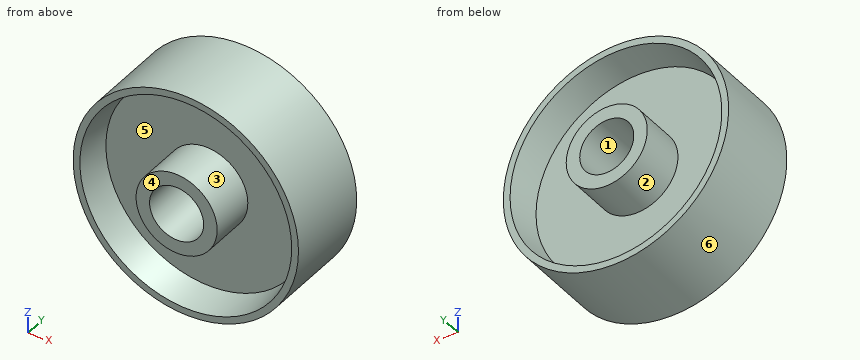
Autodesk Inventor part; units mm, degrees
ref_plane "YZ Plane" through (0, 0, 0) normal (1, 0, 0) x (0, 1, 0)
ref_plane "XZ Plane" through (0, 0, 0) normal (0, 1, 0) x (-1, 0, 0)
ref_plane "XY Plane" through (0, 0, 0) normal (0, 0, 1) x (1, 0, 0)
sketch "Sketch1" plane through (0, 0, 0) normal (0, 0, 1) x (1, 0, 0)
  line L0 (0, 40) -> (0, -30)
  line L1 (8.2, 0) -> (61.4, 0)
  line L2 (12, 25) -> (12, -25)
  line L3 (12, 25) -> (18, 25)
  line L4 (18, 25) -> (18, 5)
  line L5 (18, 5) -> (45, 5)
  line L6 (47, 19) -> (50, 19)
  line L7 (50, 19) -> (50, -19)
  line L8 (50, -19) -> (47, -19)
  line L9 (47, -19) -> (45, -5)
  line L10 (45, -5) -> (18, -5)
  line L11 (18, -5) -> (18, -25)
  line L12 (18, -25) -> (12, -25)
  line L13 (45, 5) -> (47, 19)
  dimension "d0" = 50
  dimension "d1" = 24
  dimension "d2" = 36
  dimension "d3" = 100
  dimension "d4" = 3
  dimension "d5" = 10
  dimension "d6" = 5
  dimension "d7" = 38
revolve "Revolution1" add sketch "Sketch1" angle 360 about axis through (0, 0, 0) along (0, -1, 0)
properties part number "Wheel" material "Thermoplastic Resin"
Design review of the part built by this model. Coordinates are the model's own, in mm. Face numbers are marked on the shaded views. A direction names the side the tool comes from. Round coordinates to 2 decimals unless told otherwise and drop trailing zeros. Write each loop counter-clockwise with the first axis right and the second up, starting at its lowest first coordinate (ties: lowest second). Pieces come first, ordered by that corner, then holes. Notation, with made-up numbers: (8, 82) - (43, 82) arc R27 ccw to (43, 100) - close; hole circle Ø3 at (53.5, 20.5). An arc over 180 degrees is marked (long way). Return JSON: item names as keys, results as strings. Group by question number.
Item 1: For probe 1 along Z at (x, y) = (0, 4.5); probe 2 along X at (y, z) = (-18.5, 1.5); probe 3 along X at (y, z) = (20.5, 0.5), list the stretches that pass through material, from the lowest coordinate up. Write a range as [from, to].
Item 2: We need section D-D on y = 22.5. Write out the cut boundary in (x, z), and give its area (3 significant figures).
Item 3: Insertion check: P1, Ø3, axis at x = 38.5, z = -36.5, coming from the +Y side; P2, Ø10, axis at x = -11.5, y = 7, coming from the -Z side; P3, Ø8, axis at x = -38.5, z = -36.5, coming from the +Y side; P4, Ø8, axis at x = 17.5, z = -24, coming from the -Y side. Each pin has a flat end and moves straight along its axis. Give the tip position at first contact, or say it passes through.
Item 4: We need section B-B on x = 0. Write out the cut boundary in (y, z).
Item 5: We need section A-A on z = 0. Write out the cut boundary in (x, y), and give its area (3 significant figures).
Item 6: Machinability: for the marked faces 1, 2 and 3, which of the approach directions +Z, -Z, +X, -X, +Y, -Y give a long, thin tool a straight path to every point of the face, cutting with its end or side? Answer none if there is none.
Item 7: We need section C-C on y = 12. Write out the cut boundary in (x, z).
Item 8: The part is to be moulded in two halves that separate along X. For the marked faces 4, 5 and 6, say which applies: pulls with the +X half, pulls with the -X half, needs draft (parallel to the pull), parting line crosses it, or undercut.
Model answer:
{
 "1": {"probe 1": "z = [-50, -12], [12, 50]", "probe 2": "x = [-49.98, -46.9], [-17.94, -11.91], [11.91, 17.94], [46.9, 49.98]", "probe 3": "x = [-17.99, -11.99], [11.99, 17.99]"},
 "2": {"outline": "circle Ø36 at (0, 0); hole circle Ø24 at (0, 0)", "area": "565 mm²"},
 "3": {"P1": "passes through", "P2": "stops at z = -49.58", "P3": "stops at y = 19", "P4": "stops at y = -5"},
 "4": {"outline": "(-25, -18) - (-5, -18) - (-5, -45) - (-19, -47) - (-19, -50) - (19, -50) - (19, -47) - (5, -45) - (5, -18) - (25, -18) - (25, -12) - (-25, -12) - close; (-25, 12) - (25, 12) - (25, 18) - (5, 18) - (5, 45) - (19, 47) - (19, 50) - (-19, 50) - (-19, 47) - (-5, 45) - (-5, 18) - (-25, 18) - close"},
 "5": {"outline": "(-50, -19) - (-47, -19) - (-45, -5) - (-18, -5) - (-18, -25) - (-12, -25) - (-12, 25) - (-18, 25) - (-18, 5) - (-45, 5) - (-47, 19) - (-50, 19) - close; (12, -25) - (18, -25) - (18, -5) - (45, -5) - (47, -19) - (50, -19) - (50, 19) - (47, 19) - (45, 5) - (18, 5) - (18, 25) - (12, 25) - close", "area": "1,460 mm²"},
 "6": {"face 1": "+Y, -Y", "face 2": "+Y", "face 3": "-Y"},
 "7": {"outline": "circle Ø100 at (0, 0); circle Ø36 at (0, 0); hole circle Ø92 at (0, 0); hole circle Ø24 at (0, 0)"},
 "8": {"face 4": "needs draft", "face 5": "undercut", "face 6": "parting line crosses it"}
}
